Source: CAD feature listing. Evaluate the final solid. Frame: model axes, mm. A direction names the side the tool comes from. Give positions to 0.01 mm unless a question says otherwise; leave off trailing zeros. Order: outer loops, then holes, each group sorted by start corner. A loop starts at its lowest first (then second) coordinate and runs counter-clockwise, first axis right, second up. Notation, with made-up numbers: (66.5, 24) - (116.5, 24) arc R29 ccw to (116.5, 46) - close; hole circle Ø9 at (38.25, 27). An arc over 180 degrees is marked (long way). Use CSV: the item, a comma, the result in double quotes.
```python
from build123d import *

# Parameters (mm, degrees)
SKETCH_1_R          = 9.5
EXTRUDE_1_DEPTH     = 11
SKETCH_2_R          = 10.55
CUT_EXTRUDE_1_DEPTH = 5
SKETCH_3_W          = 35
SKETCH_3_H          = 4
EXTRUDE_2_DEPTH     = 31
SKETCH_5_R          = 10.5
SKETCH_5_R_2        = 2.1
EXTRUDE_3_DEPTH     = 3.5
SKETCH_7_W          = 61.53340186
SKETCH_7_H          = 39.361856863
CUT_EXTRUDE_4_DEPTH = 56.138462075
SKETCH_8_R          = 2.1
CUT_EXTRUDE_5_DEPTH = 20
SKETCH_9_R          = 3.8
CUT_EXTRUDE_6_DEPTH = 2.2


with BuildPart() as part:
    # 草图1 → 凸台-拉伸1 (new body)
    with BuildSketch(Plane(origin=(0, 0, 0), x_dir=(1, 0, 0), z_dir=(0, 1, 0))):
        Polygon((-17.5, 0), (-17.5, -25), (17.5, -25), (17.5, 0), (17.5, 25), (-17.5, 25), align=None)
        with Locations(Location((0, 0, 0), (0, 0, 270))):
            Circle(SKETCH_1_R, mode=Mode.SUBTRACT)
    extrude(amount=EXTRUDE_1_DEPTH)

    # 草图2 → 切除-拉伸1 (cut)
    with BuildSketch(Plane(origin=(0, 11, 0), x_dir=(1, 0, 0), z_dir=(0, 1, 0))):
        with Locations(Location((0, 0, 0), (0, 0, 270))):
            Circle(SKETCH_2_R)
    cut_extrude_1 = extrude(amount=-CUT_EXTRUDE_1_DEPTH, mode=Mode.SUBTRACT)

    # 镜向1: 切除-拉伸1 across plane
    add(cut_extrude_1.mirror(Plane.ZX.offset(5.5)), mode=Mode.SUBTRACT)

    # 草图3 → 凸台-拉伸2 (add)
    with BuildSketch(Plane.XZ):
        with Locations((0, 23)):
            Rectangle(SKETCH_3_W, SKETCH_3_H)
    extrude(amount=EXTRUDE_2_DEPTH)

    # 草图5 → 凸台-拉伸3 (add)
    with BuildSketch(Plane.XZ.offset(31)):
        with BuildLine():
            Line((-17.5, 25), (-17.5, 0))
            ThreePointArc((-17.5, 0), (0, -17.5), (17.5, 0))
            Line((17.5, 0), (17.5, 25))
            Line((17.5, 25), (-17.5, 25))
        make_face()
        with Locations(Location((0, 0, 0), (0, 0, 270))):
            Circle(SKETCH_5_R, mode=Mode.SUBTRACT)
        with Locations(Location((0, 14, 0), (0, 0, 270))):
            Circle(SKETCH_5_R_2, mode=Mode.SUBTRACT)
        with Locations(Location((14, 0, 0), (0, 0, 270))):
            Circle(SKETCH_5_R_2, mode=Mode.SUBTRACT)
        with Locations(Location((0, -14, 0), (0, 0, 270))):
            Circle(SKETCH_5_R_2, mode=Mode.SUBTRACT)
        with Locations(Location((-14, 0, 0), (0, 0, 270))):
            Circle(SKETCH_5_R_2, mode=Mode.SUBTRACT)
    extrude(amount=EXTRUDE_3_DEPTH)

    # 草图7 → 切除-拉伸4 (cut, through all)
    with BuildSketch(Plane.ZY.offset(17.5)):
        with Locations((-3.514973955, -19.680928431)):
            Rectangle(SKETCH_7_W, SKETCH_7_H)
    extrude(amount=-CUT_EXTRUDE_4_DEPTH, mode=Mode.SUBTRACT)

    # 草图8 → 切除-拉伸5 (cut)
    with BuildSketch(Plane.XZ):
        with Locations(Location((-12.5, 20, 0), (0, 0, 270))):
            Circle(SKETCH_8_R)
        with Locations(Location((12.5, 20, 0), (0, 0, 90))):
            Circle(SKETCH_8_R)
        with Locations(Location((12.5, -20, 0), (0, 0, 270))):
            Circle(SKETCH_8_R)
        with Locations(Location((-12.5, -20, 0), (0, 0, 90))):
            Circle(SKETCH_8_R)
    extrude(amount=-CUT_EXTRUDE_5_DEPTH, mode=Mode.SUBTRACT)

    # 草图9 → 切除-拉伸6 (cut)
    with BuildSketch(Plane.XZ):
        with Locations(Location((-12.5, 20, 0), (0, 0, 270))):
            Circle(SKETCH_9_R)
        with Locations(Location((12.5, 20, 0), (0, 0, 90))):
            Circle(SKETCH_9_R)
        with Locations(Location((12.5, -20, 0), (0, 0, 270))):
            Circle(SKETCH_9_R)
        with Locations(Location((-12.5, -20, 0), (0, 0, 90))):
            Circle(SKETCH_9_R)
    extrude(amount=-CUT_EXTRUDE_6_DEPTH, mode=Mode.SUBTRACT)


solid = part.part
```
Item 1: Material intervals for line 1 (X direction, y = 1, z = -20); line 2 (X direction, y = 3.25, z = 0.5); line 3 (X direction, y = 8, z = 20), sorted ascending. Write a range as from..to.
Filled in:
line 1,"x = -17.5..-16.3, -8.7..8.7, 16.3..17.5"
line 2,"x = -17.5..-10.54, 10.54..17.5"
line 3,"x = -17.5..-14.6, -10.4..10.4, 14.6..17.5"
Item 2: Section B-B on y = 10. Return the cut outline in (x, z).
Filled in:
outline,"(-17.5, -25) - (17.5, -25) - (17.5, 25) - (-17.5, 25) - close; hole circle Ø4.2 at (-12.5, -20); hole circle Ø4.2 at (-12.5, 20); hole circle Ø21.1 at (0, 0); hole circle Ø4.2 at (12.5, -20); hole circle Ø4.2 at (12.5, 20)"
Item 3: First-contact query: pin 1 (6.5 mm diameter, centred on x = 2.5, z = 2.5, fed in from -Y); pin 2 (5.5 mm diameter, centred on x = 12.5, z = -20, fed in from -Y). Flat tips, straight axial feed; report the tip coordinate or a pass-through.
Filled in:
pin 1,"passes through"
pin 2,"stops at y = 2.2"
Item 4: Section C-C on z = 20. Return the cut outline in (x, y).
Filled in:
outline,"(-17.5, 0) - (-16.3, 0) - (-16.3, 2.2) - (-14.6, 2.2) - (-14.6, 11) - (-17.5, 11) - close; (-10.4, 2.2) - (-8.7, 2.2) - (-8.7, 0) - (8.7, 0) - (8.7, 2.2) - (10.4, 2.2) - (10.4, 11) - (-10.4, 11) - close; (14.6, 2.2) - (16.3, 2.2) - (16.3, 0) - (17.5, 0) - (17.5, 11) - (14.6, 11) - close"
Item 5: Section A-A on x = -12.5. Return the cut outline in (y, z), then the cut area to 3 significant figures.
Filled in:
outline,"(0, -25) - (11, -25) - (11, -22.1) - (2.2, -22.1) - (2.2, -23.8) - (0, -23.8) - close; (0, -16.2) - (2.2, -16.2) - (2.2, -17.9) - (11, -17.9) - (11, 17.9) - (2.2, 17.9) - (2.2, 16.2) - (0, 16.2) - close; (0, 23.8) - (2.2, 23.8) - (2.2, 22.1) - (11, 22.1) - (11, 25) - (0, 25) - close"
area,"443 mm2"
Item 6: Mould query, pull axis Z, two halves, no side actions, for faces 1 (the flat face through (-17.5, 6, 0)), 2 (the flat face through (-14, 2.2, 18)), 3 (the flat face through (0, 6, 25)). Classes: released by +Z, released by -Z, zero draft, split by the parting line, or undercut.
Filled in:
face 1,"zero draft"
face 2,"undercut"
face 3,"released by +Z"
Item 7: Set-up query: faces 4 (the cylindrical face through (-11.7, 6.54, -18.06)), 5 (the cylindrical face through (15.704, 1.085, -22.043)), 6 (the cylindrical face through (7.13, 8.535, -7.776)). Return all of +Z, -Z, +X, -X, +Y, -Y with unobstructed straight access to the full face (end or side cutting, diameter ignored); none if empty.
Filled in:
face 4,"+Y, -Y"
face 5,"-Y"
face 6,"+Y"
Item 8: Section D-D on x = 0. Return the cut outline in (y, z).
Filled in:
outline,"(0, -25) - (11, -25) - (11, -10.55) - (6, -10.55) - (6, -9.5) - (5, -9.5) - (5, -10.55) - (0, -10.55) - close; (0, 10.55) - (5, 10.55) - (5, 9.5) - (6, 9.5) - (6, 10.55) - (11, 10.55) - (11, 25) - (0, 25) - close"
